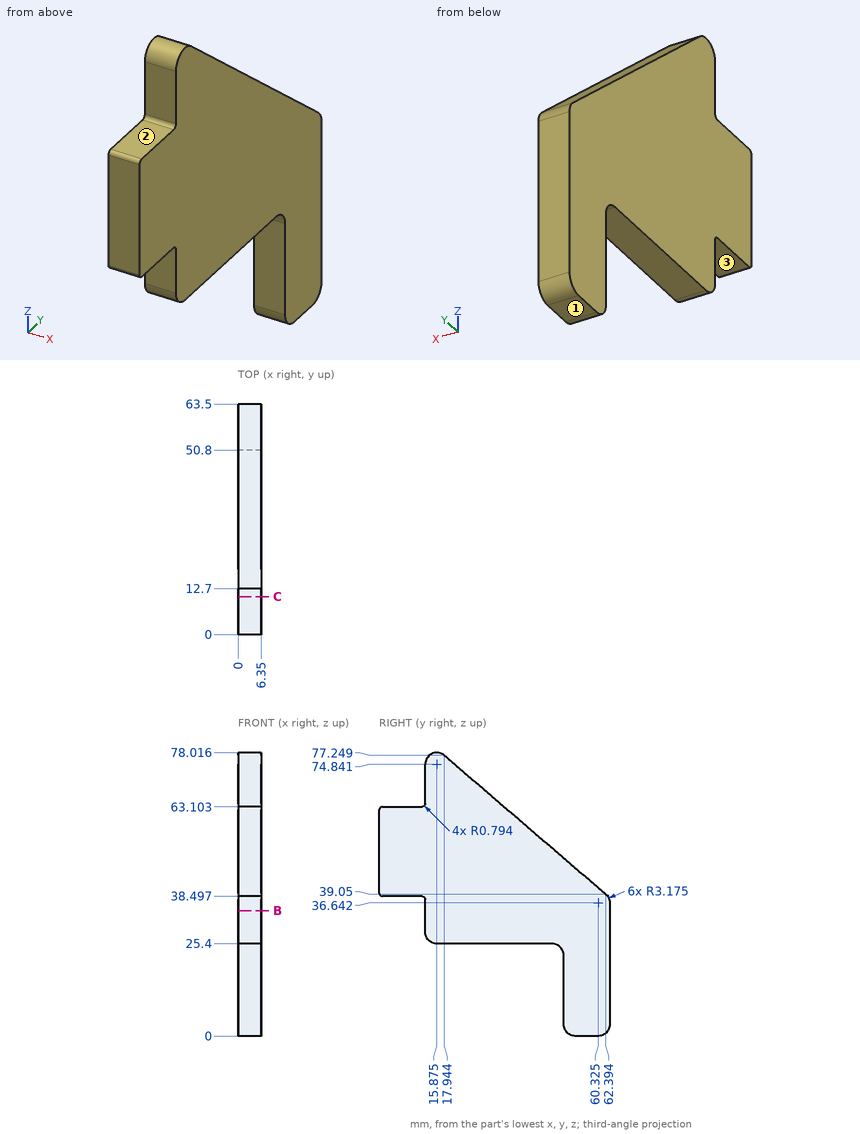
The drawing under review shows one solid part. Ordinate dimensions are in mm from its lowest x, y, z. A direction names the side the tool comes from. Coordinates: 2 decimals unless noted, no trailing zeros. Order: outer loops, then holes, each group sorted by start corner. A loop starts at its lowest first (then second) coordinate and runs counter-clockwise, first axis right, second up. Notation, with made-up numbers: M 29,81 L 39,81 A22 cw 39,104 Z; hole C -29.5,-21.5 d9. An arc over 180 degrees is marked long. Use a Markdown table: item, result.
(1) Add section C-C (y = 10.5). Give the boundary of the cut face in (x, z), then the cut area to 3 significant figures.
Worked answers:
| item | result |
|---|---|
| outline | M 0,38.5 L 6.35,38.5 L 6.35,63.1 L 0,63.1 Z |
| area | 156 mm2 |
(2) For the marked faces 1, 2 and 3, list the 3-axis set-ups (+Z, -Z, +X, -X, +Y, -Y) from which the entire face can be reached by the end or side of a thin tool; tool diameter is ignored.
Worked answers:
| item | result |
|---|---|
| face 1 | -Z, +X, -X, +Y, -Y |
| face 2 | +Z, +X, -X, -Y |
| face 3 | -Z, +X, -X, -Y |
(3) For P1, Ø2, axis at x = 4, y = 29.5, coming from the +Z side; P2, Ø1.5, axis at x = 3.5, z = 15, coming from the -Y side; P3, Ø3, axis at x = 2.5, y = 8.5, coming from the -Z side; P4, Ø8, axis at y = 37.5, z = 20, coming from the +X side, all flat-tipped, find the tip position at first contact; note any pin that passes through.
Worked answers:
| item | result |
|---|---|
| P1 | stops at z = 68.18 |
| P2 | stops at y = 50.8 |
| P3 | stops at z = 38.5 |
| P4 | passes through |
(4) Add section B-B (z = 34.5). Give the boundary of the cut face in (x, y).
Worked answers:
| item | result |
|---|---|
| outline | M 0,12.7 L 6.35,12.7 L 6.35,63.5 L 0,63.5 Z |
(5) Wall thickness on probe 1 along Y at (x, z) = (5.75, 29.5); probe 2 along Y at (x, z) = (4, 26.5); probe 3 along Z at (x, y) = (0.5, 40) (1 decimal): over which ranges is each line inside the solid? List them lowest first.
Worked answers:
| item | result |
|---|---|
| probe 1 | y = 12.7 to 63.5 |
| probe 2 | y = 13.47 to 63.5 |
| probe 3 | z = 25.4 to 58.3 |
